Design review of the part built by this model. Coordinates are the model's own, in mm. A direction names the side the tool comes from. Round coordinates to 2 decimals unless told otherwise and drop trailing zeros. Loops run counter-clockwise (first coordinate to the right, second up) from the corner with the lowest first, then second, coordinate; pieces in that order, holes last. Notation, with made-up numbers: M 57.25,87 L 83.25,87 A36 ccw 83.25,124 Z; hole C 88.25,43.5 d9. An arc over 180 degrees is marked long. Answer as CSV lines item,"result". Start each with the question number.
from build123d import *

# Parameters (mm, degrees)
SKETCH1_W               = 152.4
SKETCH1_H               = 152.4
BOSS_EXTRUDE1_DEPTH     = 35
SKETCH2_R               = 7.55
CUT_EXTRUDE1_DEPTH      = 114.304368848
CHAMFER1_SIZE           = 18
CUT_EXTRUDE2_REACH      = 175.946
CUT_EXTRUDE2_END_RADIUS = 7.55
SKETCH4_R               = 5
SKETCH5_W               = 127
SKETCH5_H               = 127
CUT_EXTRUDE3_DEPTH      = 25
CHAMFER3_SIZE           = 1


with BuildPart() as part:
    # Sketch1 → Boss-Extrude1 (new body)
    with BuildSketch(Plane(origin=(0, 0, 0), x_dir=(1, 0, 0), z_dir=(0, 1, 0))):
        Rectangle(SKETCH1_W, SKETCH1_H)
    extrude(amount=BOSS_EXTRUDE1_DEPTH)

    # Sketch2 → Cut-Extrude1 (cut, through all)
    with BuildSketch(Plane(origin=(0, 35, 0), x_dir=(1, 0, 0), z_dir=(0, 1, 0))):
        with Locations(Location((0, 0, 0), (0, 0, 270))):
            Circle(SKETCH2_R)
    extrude(amount=-CUT_EXTRUDE1_DEPTH, mode=Mode.SUBTRACT)

    # Chamfer1
    chamfer1_edges = [part.edges().sort_by_distance(p)[0] for p in [
        (76.2, 35, 0),
        (0, 35, -76.2),
        (-76.2, 35, 0),
        (0, 35, 76.2),
    ]]
    chamfer(chamfer1_edges, length=CHAMFER1_SIZE)

    # Cut-Extrude2: up to this cylinder (the profile starts outside it)
    cut_extrude2_end = Plane(origin=(0, 3, 0), z_dir=(0, 1, 0)) * Cylinder(CUT_EXTRUDE2_END_RADIUS, 367.992, mode=Mode.PRIVATE)
    # Sketch4 → Cut-Extrude2 (cut, up to the surface)
    with BuildSketch(Plane(origin=(76.2, 0, 0), x_dir=(0, 0, -1), z_dir=(1, 0, 0)), mode=Mode.PRIVATE) as cut_extrude2_sk1:
        with Locations((0, 3)):
            Circle(SKETCH4_R)
    cut_extrude2_tool1 = extrude(cut_extrude2_sk1.sketch, amount=-CUT_EXTRUDE2_REACH, mode=Mode.PRIVATE) - cut_extrude2_end
    add(cut_extrude2_tool1.solids().sort_by_distance((76.2, 3, 0))[0], mode=Mode.SUBTRACT)

    # Sketch5 → Cut-Extrude3 (cut)
    with BuildSketch(Plane.XZ):
        Rectangle(SKETCH5_W, SKETCH5_H)
    extrude(amount=-CUT_EXTRUDE3_DEPTH, mode=Mode.SUBTRACT)

    # Chamfer3
    chamfer3_edges = [part.edges().sort_by_distance(p)[0] for p in [
        (0, 35, -7.55),
    ]]
    chamfer(chamfer3_edges, length=CHAMFER3_SIZE)


solid = part.part
Item 1: Consider section A-A, the plane z = 0. Write out the cut boundary in (x, y).
Item 2: The part is to be moulded in two halves that separate along Z. For faces 1 (the face through (13, 25, 1)), 2 (the face through (-76.2, 8, 1)), 3 (the face through (-1, 8, 76.2)), say which applies: +Z half, -Z half, draft (parallel to the pull), parting line (faces both ways), or undercut.
Item 3: To check wall thickness, follow line 1 (Z direction, x = 36.5, y = 15); line 2 (Z direction, x = 70.75, y = 3). State the ranges of each line that lie inside material, in increasing order.
Item 4: Insertion check: pin 1 Ø12 at (x, z) = (-53.5, 9) entering from -Y; pin 2 Ø24 at (x, z) = (0, 0) entering from +Y; pin 3 Ø10 at (y, z) = (26, 28.5) entering from +X; pin 4 Ø1.5 at (y, z) = (23, -31.5) entering from +X. Each pin has a flat end and moves straight along its axis. Give the tip position at first contact, or say it passes through.
Item 5: Consider section D-D, the plane x = -25. Write out the cut boundary in (y, z), then the cut area to 4 significant figures.
Item 6: Tool access review of faces 4 (the face through (-63.5, 12, -1)), 5 (the face through (-14, 35, -1)), 6 (the face through (70, 8, 0)): name each direction out of +Z, -Z, +X, -X, +Y, -Y from which nothing blocks a thin tool from reaching the whole face with its end or side.
Item 7: Consider section B-B, the plane x = 0. Write out the cut boundary in (y, z).
Item 8: Consider section C-C, the plane y = 15. Write out the cut boundary in (x, z).
Found:
1,outline,"M -76.2,0 L -63.5,0 L -63.5,25 L -7.55,25 L -7.55,34 L -8.55,35 L -58.2,35 L -76.2,17 Z; M 7.55,25 L 63.5,25 L 63.5,8 L 76.2,8 L 76.2,17 L 58.2,35 L 8.55,35 L 7.55,34 Z"
2,face 1,"undercut"
2,face 2,"draft"
2,face 3,"+Z half"
3,line 1,"z = -76.2 to -63.5, 63.5 to 76.2"
3,line 2,"z = -76.2 to -5, 5 to 76.2"
4,pin 1,"stops at y = 25"
4,pin 2,"stops at y = 35"
4,pin 3,"stops at x = 72.2"
4,pin 4,"stops at x = 70.95"
5,outline,"M 0,-76.2 L 17,-76.2 L 35,-58.2 L 35,58.2 L 17,76.2 L 0,76.2 L 0,63.5 L 25,63.5 L 25,-63.5 L 0,-63.5 Z"
5,area,"1,835 mm^2"
6,face 4,"-Y"
6,face 5,"+Z, -Z, +X, -X, +Y"
6,face 6,"+X"
7,outline,"M 0,-76.2 L 17,-76.2 L 35,-58.2 L 35,-8.55 L 34,-7.55 L 25,-7.55 L 25,-63.5 L 0,-63.5 Z; M 0,63.5 L 25,63.5 L 25,7.55 L 34,7.55 L 35,8.55 L 35,58.2 L 17,76.2 L 0,76.2 Z"
8,outline,"M -76.2,-76.2 L 76.2,-76.2 L 76.2,76.2 L -76.2,76.2 Z; hole M -63.5,-63.5 L 63.5,-63.5 L 63.5,63.5 L -63.5,63.5 Z"
